The model under review builds one solid part; all positions refer to its coordinate system, in mm. A direction names the side the tool comes from. Give positions to 0.01 mm unless a question says otherwise; leave off trailing zeros. Write each loop counter-clockwise with the first axis right and the second up, starting at its lowest first coordinate (ties: lowest second). Pieces come first, ordered by that corner, then holes. Notation, with made-up numbers: M -7,-39 L -1,-39 A16 ccw -1,-32 Z; hole C -0.75,82.25 d2. An arc over 180 degrees is marked long. Write each question's results on one line, items separated by ' | '. Start each with the question number.
from build123d import *

# Parameters (mm, degrees)
F0_R     = 0.75
F0_R_2   = 1.5
F1_DEPTH = 1
F3_DEPTH = 11.48
F4_R     = 0.75
F5_DEPTH = 70
F6_R     = 0.75
F7_DEPTH = 70


with BuildPart() as f1:
    # F0 (on Top) → F1 (new body, symmetric)
    with BuildSketch(Plane.XY):
        with BuildLine():
            Line((-5.74, -35), (5.74, -35))
            Line((5.74, -35), (5.74, 35))
            ThreePointArc((5.74, 35), (0, 40.74), (-5.74, 35))
            Line((-5.74, 35), (-5.74, -35))
        make_face()
        with Locations((-2.87, 37.87)):
            Circle(F0_R, mode=Mode.SUBTRACT)
        with Locations((0, 37.87)):
            Circle(F0_R_2, mode=Mode.SUBTRACT)
        with Locations((2.87, 37.87)):
            Circle(F0_R, mode=Mode.SUBTRACT)
    extrude(amount=F1_DEPTH, both=True)

    # F2 (on face) → F3 (join)
    with BuildSketch(Plane.YZ.offset(5.74)):
        Polygon((32, 1), (35, 1), (35, 5), align=None)
        Polygon((32, -5), (32, -1), (29, -1), align=None)
        Polygon((26, 1), (29, 1), (29, 5), align=None)
        Polygon((26, -5), (26, -1), (23, -1), align=None)
        Polygon((20, 1), (23, 1), (23, 5), align=None)
        Polygon((20, -5), (20, -1), (17, -1), align=None)
        Polygon((14, 1), (17, 1), (17, 5), align=None)
        Polygon((14, -5), (14, -1), (11, -1), align=None)
        Polygon((8, 1), (11, 1), (11, 5), align=None)
        Polygon((8, -5), (8, -1), (5, -1), align=None)
        Polygon((2, 1), (5, 1), (5, 5), align=None)
        Polygon((2, -5), (2, -1), (-1, -1), align=None)
        Polygon((-4, 1), (-1, 1), (-1, 5), align=None)
        Polygon((-4, -5), (-4, -1), (-7, -1), align=None)
        Polygon((-10, 1), (-7, 1), (-7, 5), align=None)
        Polygon((-10, -5), (-10, -1), (-13, -1), align=None)
        Polygon((-16, 1), (-13, 1), (-13, 5), align=None)
        Polygon((-16, -5), (-16, -1), (-19, -1), align=None)
        Polygon((-22, 1), (-19, 1), (-19, 5), align=None)
        Polygon((-22, -5), (-22, -1), (-25, -1), align=None)
        Polygon((-28, 1), (-25, 1), (-25, 5), align=None)
        Polygon((-28, -5), (-28, -1), (-31, -1), align=None)
    extrude(amount=-F3_DEPTH)

    # F4 (on face) → F5 (cut)
    with BuildSketch(Plane(origin=(0, 35, 0), x_dir=(-1, 0, 0), z_dir=(0, 1, 0))):
        with Locations((0, 3)):
            Circle(F4_R)
    extrude(amount=-F5_DEPTH, mode=Mode.SUBTRACT)

    # F6 (on face) → F7 (cut)
    with BuildSketch(Plane(origin=(0, 32, 0), x_dir=(-1, 0, 0), z_dir=(0, 1, 0))):
        with Locations((0, -3)):
            Circle(F6_R)
    extrude(amount=-F7_DEPTH, mode=Mode.SUBTRACT)


solid = f1.part
(1) Machinability: for faces 5 (the flat face through (0, -5, 1)), 6 (the flat face through (0, 14, -4)), 7 (the flat face through (0, -35, 0)), which of the approach directions +Z, -Z, +X, -X, +Y, -Y give a long, thin tool a straight path to every point of the face, cutting with its end or side? Answer none if there is none.
(2) Draft analysis for pull direction Z (two halves, no side actions). For faces 1 (the cylindrical face through (0.098, 7.169, -2.256)), 2 (the flat face through (-5.74, 0, 0)), 3 (the flat face through (0.08, 11.81, -2.08)), 4 (the cylindrical face through (0.098, -28.831, -2.256)), state which applies: pulls with the +Z half, pulls with the -Z half, needs draft (parallel to the pull), parting line crosses it, or undercut.
(3) Clearance check with flat-ended pins moving along their axes: P1, Ø6, axis at x = 2.5, y = -2, coming from the +Z side; P2, Ø2.5, axis at x = -2, y = 21, coming from the -Z side; P3, Ø3, axis at x = 1, y = -33, coming from the -Z side; P4, Ø0.9, axis at x = 0, z = -3, coming from the +Y side. State where each tip first meets the part, or that it passes through.
(4) Wall thickness on L1, parallel to X at y = -11.45, z = -3; L2, parallel to Z at x = 0, y = -2; L3, parallel to Y at x = -1.25, z = 0.5: over which ranges is each line inside the solid? List them lowest first.
(5) Add section A-A (y = 37.87). State the section outline as (x, z) points.
(6) Add section B-B (z = -3). Give the number of separate pieces and of enclosed holes in the cut face, then the cut area to 3 significant figures.
Calculated:
1) face 5: +Z, +X, -X | face 6: -Z, +X, -X | face 7: +Z, -Z, +X, -X, -Y
2) face 1: undercut | face 2: needs draft | face 3: pulls with the -Z half | face 4: undercut
3) P1: stops at z = 5 | P2: stops at z = -5 | P3: stops at z = -1 | P4: passes through
4) L1: x = -5.74 to -0.75, 0.75 to 5.74 | L2: z = -1 to 2.25 | L3: y = -35 to 37.04, 38.7 to 40.6
5) outline: M -4.97,-1 L -3.62,-1 L -3.62,1 L -4.97,1 Z; M -2.12,-1 L -1.5,-1 L -1.5,1 L -2.12,1 Z; M 1.5,-1 L 2.12,-1 L 2.12,1 L 1.5,1 Z; M 3.62,-1 L 4.97,-1 L 4.97,1 L 3.62,1 Z
6) separate pieces: 22 | enclosed holes: 0 | area: 165 mm²
